Source: three-view drawing plus pictorial views. Frame: mm from the lowest corner of the part. Give positions to 0.01 mm unless a question says otherwise; leave off trailing zeros. Write each loop counter-clockwise with the first axis right and the second up, starting at its lowest first coordinate (ties: lowest second). Pieces come first, ordered by that corner, then holes.
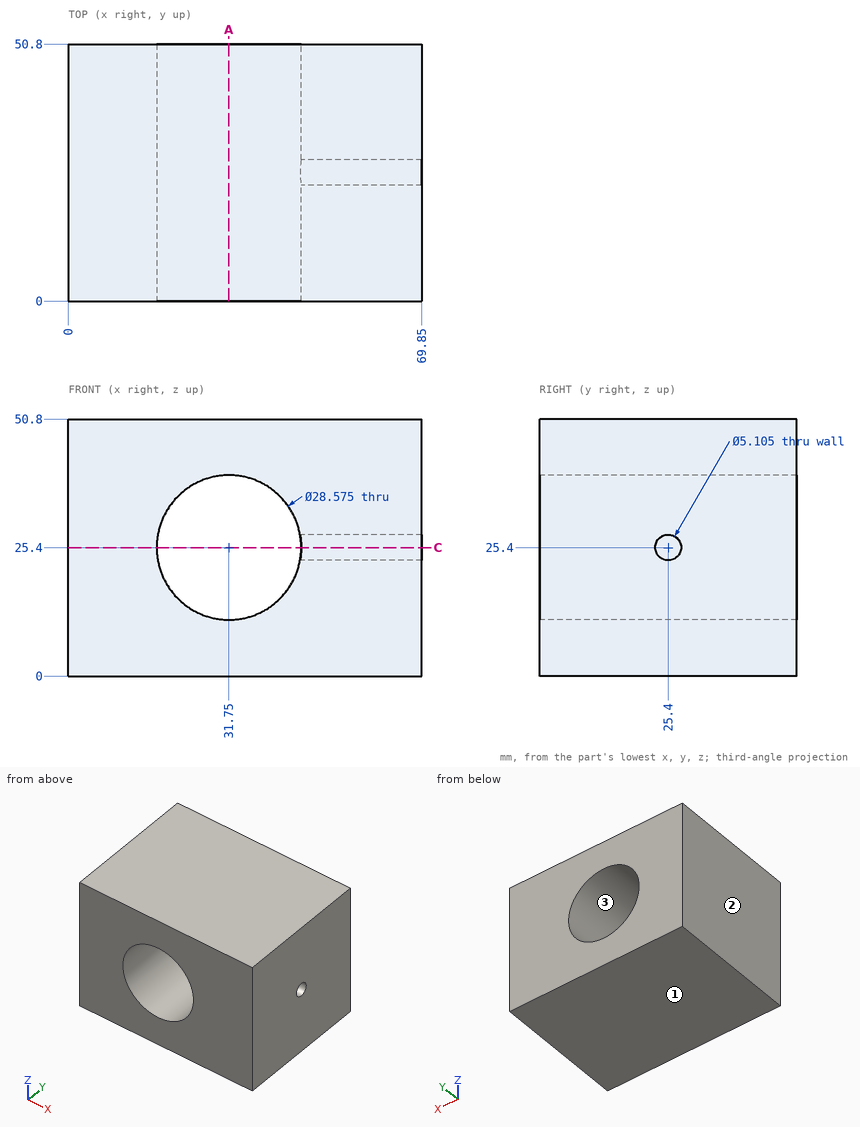
Q1. Pull-direction query (Z, two-part tool) for the marked faces 1, 2 and 3; classes: released by +Z, released by -Z, zero draft, split by the parting line, or undercut.
Filled sheet:
face 1: released by -Z
face 2: zero draft
face 3: undercut
Q2. Ray query, line 1 along Y through (x, z) = (59.25, 25.4); line 2 along Z through (x, y) = (31, 25); line 3 along Y through (x, z) = (49.5, 23.5) (1 decimal). Return the intervals inside material, ascending.
Filled sheet:
line 1: y = 0 to 22.85, 27.95 to 50.8
line 2: z = 0 to 11.13, 39.67 to 50.8
line 3: y = 0 to 23.7, 27.1 to 50.8
Q3. Section A-A on x = 31.75. Output: boundary loops of the cut face in (y, z), plus the area to 3 significant figures.
Filled sheet:
outline: (0, 0) - (50.8, 0) - (50.8, 11.11) - (0, 11.11) - close; (0, 39.69) - (50.8, 39.69) - (50.8, 50.8) - (0, 50.8) - close
area: 1,130 mm2
Q4. Section C-C on z = 25.4. Output: boundary loops of the cut face in (x, y), plus the area to 4 significant figures.
Filled sheet:
outline: (0, 0) - (17.46, 0) - (17.46, 50.8) - (0, 50.8) - close; (46.04, 0) - (69.85, 0) - (69.85, 22.85) - (46.04, 22.85) - close; (46.04, 27.95) - (69.85, 27.95) - (69.85, 50.8) - (46.04, 50.8) - close
area: 1,975 mm2
